Geometry: final body of the model. Coordinates: model frame, mm. A direction names the side the tool comes from. Coordinates: 2 decimals unless noted, no trailing zeros. Write each loop counter-clockwise with the first axis right and the second up, starting at its lowest first coordinate (ties: lowest second). Pieces come first, ordered by that corner, then holes. Notation, with made-up numbers: (-36, 52) -> (6, 52) arc R28 ccw to (6, 87) -> close; hole circle Ø2 at (-11, -9). An arc over 180 degrees is marked (long way). Answer as a JSON object with one key per item and string values. Group by question number.
```python
from build123d import *

# Parameters (mm, degrees)
SKETCH_1_W             = 77.5
SKETCH_1_H             = 45
SKETCH_1_W_2           = 71.5
SKETCH_1_H_2           = 39
EXTRUDE_1_DEPTH        = 3
SKETCH_2_W             = 3
SKETCH_2_H             = 3
EXTRUDE_2_DEPTH        = 40
SKETCH_3_W             = 3
SKETCH_3_H             = 3
EXTRUDE_3_DEPTH        = 40
EXTRUDE_4_DEPTH        = 2
EXTRUDE_4_DEPTH_BACK   = 2
EXTRUDE_4_2_DEPTH      = 2
EXTRUDE_4_2_DEPTH_BACK = 2
SKETCH_5_W             = 65.5
SKETCH_5_H             = 6
EXTRUDE_5_DEPTH        = 3
SKETCH_6_W             = 65.5
SKETCH_6_H             = 6
EXTRUDE_6_DEPTH        = 3
SKETCH_7_R             = 1.5
CUT_EXTRUDE_1_DEPTH    = 5
CHAMFER_1_SIZE         = 0.5
CHAMFER_2_SIZE         = 0.5
CHAMFER_3_SIZE         = 2
CHAMFER_4_SIZE         = 2
EXTRUDE_7_DEPTH        = 6
MIRROR_2_COPY_1_DEPTH  = 6


with BuildPart() as part:
    # Sketch 1 → Extrude 1 (new body)
    with BuildSketch(Plane.XY):
        Rectangle(SKETCH_1_W, SKETCH_1_H)
        Rectangle(SKETCH_1_W_2, SKETCH_1_H_2, mode=Mode.SUBTRACT)
    extrude(amount=EXTRUDE_1_DEPTH)

    # Sketch 2 → Extrude 2 (add)
    with BuildSketch(Plane.XY.offset(3)):
        with Locations((37.25, 21)):
            Rectangle(SKETCH_2_W, SKETCH_2_H)
        with Locations((-37.25, 21)):
            Rectangle(SKETCH_2_W, SKETCH_2_H)
        with Locations((-37.25, -21)):
            Rectangle(SKETCH_2_W, SKETCH_2_H)
        with Locations((37.25, -21)):
            Rectangle(SKETCH_2_W, SKETCH_2_H)
    extrude(amount=EXTRUDE_2_DEPTH)

    # Sketch 3 → Extrude 3 (add)
    with BuildSketch(Plane.XY.offset(3)):
        with Locations((-37.25, -18)):
            Rectangle(SKETCH_3_W, SKETCH_3_H)
        with Locations((-34.25, -21)):
            Rectangle(SKETCH_3_W, SKETCH_3_H)
        with Locations((34.25, -21)):
            Rectangle(SKETCH_3_W, SKETCH_3_H)
        with Locations((37.25, -18)):
            Rectangle(SKETCH_3_W, SKETCH_3_H)
        with Locations((37.25, 18)):
            Rectangle(SKETCH_3_W, SKETCH_3_H)
        with Locations((34.25, 21)):
            Rectangle(SKETCH_3_W, SKETCH_3_H)
        with Locations((-34.25, 21)):
            Rectangle(SKETCH_3_W, SKETCH_3_H)
        with Locations((-37.25, 18)):
            Rectangle(SKETCH_3_W, SKETCH_3_H)
    extrude(amount=EXTRUDE_3_DEPTH)

    # Sketch 5 → Extrude 5 (add)
    with BuildSketch(Plane(origin=(0, 22.5, 0), x_dir=(1, 0, 0), z_dir=(0, 1, 0))):
        with Locations((0, -6)):
            Rectangle(SKETCH_5_W, SKETCH_5_H)
    extrude(amount=-EXTRUDE_5_DEPTH)


with BuildPart() as body_2:
    # Sketch 4 → Extrude 4 (new, two sides: drawn at the far end of the back side and taken through both)
    with BuildSketch(Plane.XY.offset(43).offset(-EXTRUDE_4_DEPTH_BACK)):
        Polygon((38.75, 22.5), (53.75, 22.5), (53.75, -22.5), (38.75, -22.5), (38.75, -16.5), (39.5, -16.5), (39.5, 16.5), (38.75, 16.5), align=None)
    extrude(amount=EXTRUDE_4_DEPTH + EXTRUDE_4_DEPTH_BACK)


with BuildPart() as body_3:
    # Sketch 4 → Extrude 4 2 (new, two sides: drawn at the far end of the back side and taken through both)
    with BuildSketch(Plane.XY.offset(43).offset(-EXTRUDE_4_2_DEPTH_BACK)):
        Polygon((-38.75, -16.5), (-38.75, -22.5), (-53.75, -22.5), (-53.75, 22.5), (-38.75, 22.5), (-38.75, 16.5), (-39.5, 16.5), (-39.5, -16.5), align=None)
    extrude(amount=EXTRUDE_4_2_DEPTH + EXTRUDE_4_2_DEPTH_BACK)


with BuildPart() as body_4:
    # Sketch 6 → Extrude 6 (new body)
    with BuildSketch(Plane.XZ.offset(22.5)):
        with Locations((0, 6)):
            Rectangle(SKETCH_6_W, SKETCH_6_H)
    extrude(amount=-EXTRUDE_6_DEPTH)


with BuildPart() as cut_extrude_1_tool:
    # Sketch 7 → Cut-Extrude 1 (new body)
    with BuildSketch(Plane.XY.offset(45)):
        with Locations((-46, 0)):
            Circle(SKETCH_7_R)
        with Locations((46, 0)):
            Circle(SKETCH_7_R)
    extrude(amount=-CUT_EXTRUDE_1_DEPTH)


with BuildPart() as body_2_1:
    add(body_2.part)

    # Cut-Extrude 1: cut by cut_extrude_1_tool
    add(cut_extrude_1_tool.part, mode=Mode.SUBTRACT)

    # Chamfer 2
    chamfer_2_edges = [body_2_1.edges().sort_by_distance(p)[0] for p in [
        (44.5, 0, 45),
    ]]
    chamfer(chamfer_2_edges, length=CHAMFER_2_SIZE)

    # Chamfer 3
    chamfer_3_edges = [body_2_1.edges().sort_by_distance(p)[0] for p in [
        (53.75, 22.5, 43),
        (53.75, -22.5, 43),
    ]]
    chamfer(chamfer_3_edges, length=CHAMFER_3_SIZE)


with BuildPart() as body_3_1:
    add(body_3.part)

    # Cut-Extrude 1: cut by cut_extrude_1_tool
    add(cut_extrude_1_tool.part, mode=Mode.SUBTRACT)

    # Chamfer 1
    chamfer_1_edges = [body_3_1.edges().sort_by_distance(p)[0] for p in [
        (-47.5, 0, 45),
    ]]
    chamfer(chamfer_1_edges, length=CHAMFER_1_SIZE)


with BuildPart() as part_1:
    add(part.part)

    # Combine 1: union body 3
    add(body_3_1.part)


with BuildPart() as body_4_1:
    add(body_4.part)

    # Combine 2: union part
    add(part_1.part)


with BuildPart() as body_2_2:
    add(body_2_1.part)

    # Combine 3: union body 4
    add(body_4_1.part)

    # Chamfer 4
    chamfer_4_edges = [body_2_2.edges().sort_by_distance(p)[0] for p in [
        (-53.75, 22.5, 43),
        (-53.75, -22.5, 43),
    ]]
    chamfer(chamfer_4_edges, length=CHAMFER_4_SIZE)

    # Sketch 8 → Extrude 7 (add)
    with BuildSketch(Plane(origin=(0, 22.5, 0), x_dir=(1, 0, 0), z_dir=(0, 1, 0))):
        Polygon((48.75, -41), (38.75, -26), (38.75, -41), align=None)
    extrude_7 = extrude(amount=-EXTRUDE_7_DEPTH)

    # Mirror 1: Extrude 7 across plane
    add(extrude_7.mirror(Plane(origin=(0, 0, 0), x_dir=(0, 0, 1), z_dir=(1, 0, 0))))

    # Mirror 2: Extrude 7 across plane
    add(extrude_7.mirror(Plane.ZX))

    # Mirror 2 copy 1 sketch → Mirror 2 copy 1 (add)
    with BuildSketch(Plane(origin=(0, -22.5, 0), x_dir=(-1, 0, 0), z_dir=(0, -1, 0))):
        Polygon((48.75, -41), (38.75, -26), (38.75, -41), align=None)
    extrude(amount=-MIRROR_2_COPY_1_DEPTH)


solid = body_2_2.part
```
Item 1: Mould query, pull axis Y, two halves, no side actions, for faces 1 (the flat face through (-37, 0, 3)), 2 (the flat face through (38.75, -0.1, 0.4)), 3 (the flat face through (52.74, -21.51, 42.97)). Classes: +Y half, -Y half, draft (parallel to the pull), parting line (faces both ways), or undercut.
Item 2: Set-up query: faces 4 (the flat face through (-49, 0, 45)), 5 (the flat face through (-38.75, -0.1, 0.4)), 6 (the flat face through (32.75, 21, 26)), 7 (the flat face through (-53.75, 0, 43)), 8 (the flat face through (0, 19.5, 7)). Return all of +Z, -Z, +X, -X, +Y, -Y with unobstructed straight access to the full face (end or side cutting, diameter ignored); none if empty.
Item 3: Section C-C on x = -3. Output: boundary loops of the cut face in (y, z).
Item 4: Section A-A on y = 12. Output: boundary loops of the cut face in (x, z).
Item 5: Section D-D on z = 8. Output: boundary loops of the cut face in (x, y).
Item 6: Contact query for flat-ended pins moving along their axis: pin 1 (0.9 mm diameter, centred on y = 20.5, z = 24, fed in from -X); pin 2 (2.5 mm diameter, centred on x = -46, y = 0, fed in from +Z); pin 3 (2.5 mm diameter, centred on x = 37, y = 2, fed in from +Z); pin 4 (0.9 mm diameter, centred on y = -21, z = 31, fed in from +X). Output: stop coordinate, or through.
Item 7: Ray query, L1, parallel to Y at x = -37, z = 30; L2, parallel to Y at x = -46, z = 43; L3, parallel to Z at x = 46, y = -9.5. Return the intervals inside material, ascending. Write a range as [from, to].
Item 8: Section B-B on z = 22.5. Output: boundary loops of the cut face in (x, y), then the cut area to 3 significant figures.
Answer sheet:
{
 "1": {"face 1": "undercut", "face 2": "draft", "face 3": "-Y half"},
 "2": {"face 4": "+Z, +X, -X, +Y, -Y", "face 5": "-Z, -X, +Y, -Y", "face 6": "+Z, +Y, -Y", "face 7": "+Z, -Z, -X, +Y, -Y", "face 8": "+Z, -Z"},
 "3": {"outline": "(-22.5, 0) -> (-19.5, 0) -> (-19.5, 9) -> (-22.5, 9) -> close; (19.5, 0) -> (22.5, 0) -> (22.5, 9) -> (19.5, 9) -> close"},
 "4": {"outline": "(-53.75, 41) -> (-39.5, 41) -> (-39.5, 45) -> (-53.75, 45) -> close; (-38.75, 0) -> (-35.75, 0) -> (-35.75, 3) -> (-38.75, 3) -> close; (35.75, 0) -> (38.75, 0) -> (38.75, 3) -> (35.75, 3) -> close; (39.5, 41) -> (53.75, 41) -> (53.75, 45) -> (39.5, 45) -> close"},
 "5": {"outline": "(-38.75, -22.5) -> (38.75, -22.5) -> (38.75, -16.5) -> (35.75, -16.5) -> (35.75, -19.5) -> (-35.75, -19.5) -> (-35.75, -16.5) -> (-38.75, -16.5) -> close; (-38.75, 16.5) -> (-35.75, 16.5) -> (-35.75, 19.5) -> (35.75, 19.5) -> (35.75, 16.5) -> (38.75, 16.5) -> (38.75, 22.5) -> (-38.75, 22.5) -> close"},
 "6": {"pin 1": "stops at x = -38.75", "pin 2": "passes through", "pin 3": "stops at z = 3", "pin 4": "stops at x = 42.38"},
 "7": {"L1": "y = [-22.5, -16.5], [16.5, 22.5]", "L2": "y = [-22.5, -1.5], [1.5, 22.5]", "L3": "z = [41, 45]"},
 "8": {"outline": "(-38.75, -22.5) -> (-32.75, -22.5) -> (-32.75, -19.5) -> (-35.75, -19.5) -> (-35.75, -16.5) -> (-38.75, -16.5) -> close; (-38.75, 16.5) -> (-35.75, 16.5) -> (-35.75, 19.5) -> (-32.75, 19.5) -> (-32.75, 22.5) -> (-38.75, 22.5) -> close; (32.75, -22.5) -> (38.75, -22.5) -> (38.75, -16.5) -> (35.75, -16.5) -> (35.75, -19.5) -> (32.75, -19.5) -> close; (32.75, 19.5) -> (35.75, 19.5) -> (35.75, 16.5) -> (38.75, 16.5) -> (38.75, 22.5) -> (32.75, 22.5) -> close", "area": "108 mm^2"}
}
